Read the model definition and answer for the solid it produces. Units are mm, in the model's axes. A direction names the side the tool comes from. Give positions to 0.01 mm unless a question says otherwise; leave off trailing zeros. Order: outer loops, then holes, each group sorted by start corner. A loop starts at its lowest first (then second) coordinate and runs counter-clockwise, first axis right, second up.
Item 1: The mould has two halves that part along X. Classify faces 1 (the face through (45.03, -4.48, -1.61)), 2 (the face through (-48, -1, 0)), 3 (the face through (-44, 1, -1)), 4 (the face through (36, 8, 22)): +X half, -X half, draft (parallel to the pull), parting line (faces both ways), or undercut.
Item 2: Which of the six approach directions +Z, -Z, +X, -X, +Y, -Y give full straight-line access (tool end or side, diameter ignored) to faces 5 (the face through (43, -1, 6)), 6 (the face through (0, 10, 20)), 7 (the face through (44, 1, 1)), 8 (the face through (37, 1, -14))?
Item 3: Find the intervals of material crossed by line 1 along X through (y, z) = (-2, 0); line 2 along X through (y, z) = (-3.25, 0); line 3 along Z through (x, y) = (42.5, -1.5), in increasing order.
Item 4: Given pin 1 Ø4 at (x, z) = (42.5, 0) entering from +Y; pin 2 Ø2 at (x, z) = (-15, 11) entering from -Y; pin 3 Ø4.5 at (x, y) = (-44, -1) entering from +Z, each flat-ended and moving along its own axis, determine where each tip first touches the part or whether it passes through.
Item 5: A cutting plane is placed at B-B (x = -42.5). Write down the section's boundary in (y, z).
Item 6: A cutting plane is placed at D-D (z = 11). Write down the section's boundary in (x, y).
Item 7: A cutting plane is placed at C-C (x = 2). Write down the section's boundary in (y, z).
Item 8: A cutting plane is placed at A-A (z = 0). Write down the section's boundary in (x, y), plus the area to 3 significant figures.
from build123d import *

# Parameters (mm, degrees)
CROQUIS1_W                     = 76
CROQUIS1_H                     = 46
CROQUIS1_W_2                   = 70
CROQUIS1_H_2                   = 40
SALIENTE_EXTRUIR1_DEPTH        = 20
CROQUIS2_W                     = 76
CROQUIS2_H                     = 46
SALIENTE_EXTRUIR2_DEPTH        = 3
SALIENTE_EXTRUIR3_DEPTH        = 3
SALIENTE_EXTRUIR3_DEPTH_BACK   = 4
CROQUIS3_R                     = 3
CROQUIS3_R_2                   = 1.5
SALIENTE_EXTRUIR3_2_DEPTH      = 3
SALIENTE_EXTRUIR3_2_DEPTH_BACK = 4
CROQUIS4_W                     = 12
CROQUIS4_H                     = 4
SALIENTE_EXTRUIR4_DEPTH        = 10
CROQUIS5_W                     = 12
CROQUIS5_H                     = 4
SALIENTE_EXTRUIR5_DEPTH        = 10
CORTAR_EXTRUIR1_START          = -10
CROQUIS6_R                     = 1.5
CORTAR_EXTRUIR1_DEPTH          = 10
CROQUIS7_W                     = 10
CROQUIS7_H                     = 16
CORTAR_EXTRUIR2_DEPTH          = 10
REDONDEO1_R                    = 5


with BuildPart() as part:
    # Croquis1 → Saliente-Extruir1 (new body)
    with BuildSketch(Plane(origin=(0, 0, 0), x_dir=(1, 0, 0), z_dir=(0, 1, 0))):
        Rectangle(CROQUIS1_W, CROQUIS1_H)
        Rectangle(CROQUIS1_W_2, CROQUIS1_H_2, mode=Mode.SUBTRACT)
    extrude(amount=SALIENTE_EXTRUIR1_DEPTH)

    # Croquis2 → Saliente-Extruir2 (add)
    with BuildSketch(Plane.XZ):
        Rectangle(CROQUIS2_W, CROQUIS2_H)
    extrude(amount=SALIENTE_EXTRUIR2_DEPTH)



with BuildPart() as body_2:
    # Croquis3 → Saliente-Extruir3 (new, two sides: drawn at the far end of the back side and taken through both)
    with BuildSketch(Plane.XZ.offset(3).offset(-SALIENTE_EXTRUIR3_DEPTH_BACK)):
        with Locations(Location((42.5, 0, 0), (0, 0, 270))):
            Circle(CROQUIS3_R)
        with Locations(Location((42.5, 0, 0), (0, 0, 270))):
            Circle(CROQUIS3_R_2, mode=Mode.SUBTRACT)
    extrude(amount=SALIENTE_EXTRUIR3_DEPTH + SALIENTE_EXTRUIR3_DEPTH_BACK)


with BuildPart() as body_3:
    # Croquis3 → Saliente-Extruir3 2 (new, two sides: drawn at the far end of the back side and taken through both)
    with BuildSketch(Plane.XZ.offset(3).offset(-SALIENTE_EXTRUIR3_2_DEPTH_BACK)):
        with Locations(Location((-42.5, 0, 0), (0, 0, 270))):
            Circle(CROQUIS3_R)
        with Locations(Location((-42.5, 0, 0), (0, 0, 270))):
            Circle(CROQUIS3_R_2, mode=Mode.SUBTRACT)
    extrude(amount=SALIENTE_EXTRUIR3_2_DEPTH + SALIENTE_EXTRUIR3_2_DEPTH_BACK)


with BuildPart() as part_1:
    add(part.part)

    add(body_2.part)  # Saliente-Extruir4 merges body 2
    # Croquis4 → Saliente-Extruir4 (add)
    with BuildSketch(Plane(origin=(38, 0, 0), x_dir=(0, 0, -1), z_dir=(1, 0, 0))):
        with Locations((0, -1)):
            Rectangle(CROQUIS4_W, CROQUIS4_H)
    extrude(amount=SALIENTE_EXTRUIR4_DEPTH)


    add(body_3.part)  # Saliente-Extruir5 merges body 3
    # Croquis5 → Saliente-Extruir5 (add)
    with BuildSketch(Plane.ZY.offset(38)):
        with Locations((0, -1)):
            Rectangle(CROQUIS5_W, CROQUIS5_H)
    extrude(amount=SALIENTE_EXTRUIR5_DEPTH)

    # Croquis6 → Cortar-Extruir1 (cut)
    with BuildSketch(Plane.XZ.offset(3).offset(CORTAR_EXTRUIR1_START)):
        with Locations(Location((-42.5, 0, 0), (0, 0, 270))):
            Circle(CROQUIS6_R)
        with Locations(Location((42.5, 0, 0), (0, 0, 270))):
            Circle(CROQUIS6_R)
    extrude(amount=CORTAR_EXTRUIR1_DEPTH, mode=Mode.SUBTRACT)

    # Croquis7 → Cortar-Extruir2 (cut)
    with BuildSketch(Plane(origin=(38, 0, 0), x_dir=(0, 0, -1), z_dir=(1, 0, 0))):
        with Locations((14, 9)):
            Rectangle(CROQUIS7_W, CROQUIS7_H)
    extrude(amount=-CORTAR_EXTRUIR2_DEPTH, mode=Mode.SUBTRACT)

    # Redondeo1
    # the kernel refuses this fillet: 5 mm, written as the material it takes off along each edge
    with BuildSketch(Plane(origin=(-38, 32.5, 23), x_dir=(1, 0, 0), z_dir=(0, -1, 0)), Plane(origin=(-38, 32.5, -23), x_dir=(0, 0, 1), z_dir=(0, -1, 0)), Plane(origin=(38, -15.5, -23), x_dir=(0, 0, 1), z_dir=(0, 1, 0)), Plane(origin=(38, -15.5, 23), x_dir=(-1, 0, 0), z_dir=(0, 1, 0))) as redondeo1_piece_1:
        with BuildLine():
            CenterArc((REDONDEO1_R, -REDONDEO1_R), REDONDEO1_R, 90, 90)
            Line((0, -REDONDEO1_R), (0, 0))
            Line((0, 0), (REDONDEO1_R, 0))
        make_face()
    extrude(amount=48, mode=Mode.SUBTRACT)


solid = part_1.part
Response values:
1. face 1: undercut
1. face 2: -X half
1. face 3: draft
1. face 4: +X half
2. face 5: +Z, +X, +Y, -Y
2. face 6: +Y
2. face 7: +Z, -Z, +X, +Y
2. face 8: +X
3. line 1: x = -48 to -44, -41 to 41, 44 to 48
3. line 2: x = -45.5 to -44, -41 to -39.5, 39.5 to 41, 44 to 45.5
3. line 3: z = -6 to -1.5, 1.5 to 6
4. pin 1: stops at y = 1
4. pin 2: stops at y = -3
4. pin 3: stops at z = 6
5. outline: (-6, -3) - (-3, -3) - (-3, -6) - (1, -6) - (1, -1.5) - (-6, -1.5) - close; (-6, 1.5) - (1, 1.5) - (1, 6) - (-3, 6) - (-3, 3) - (-6, 3) - close
6. outline: (-38, -3) - (38, -3) - (38, 20) - (35, 20) - (35, 0) - (-35, 0) - (-35, 20) - (-38, 20) - close
7. outline: (-3, -23) - (20, -23) - (20, -20) - (0, -20) - (0, 20) - (20, 20) - (20, 23) - (-3, 23) - close
8. outline: (-48, -3) - (-45.5, -3) - (-45.5, -6) - (-44, -6) - (-44, 1) - (-48, 1) - close; (-41, -6) - (-39.5, -6) - (-39.5, -3) - (39.5, -3) - (39.5, -6) - (41, -6) - (41, 1) - (38, 1) - (38, 20) - (35, 20) - (35, 0) - (-35, 0) - (-35, 20) - (-38, 20) - (-38, 1) - (-41, 1) - close; (44, -6) - (45.5, -6) - (45.5, -3) - (48, -3) - (48, 1) - (44, 1) - close
8. area: 422 mm2
